Read the model definition and answer for the solid it produces. Units are mm, in the model's axes. Face numbers are marked on the shaded views. A direction names the side the tool comes from. Coordinates: 2 decimals unless noted, no trailing zeros. Loops run counter-clockwise (first coordinate to the right, second up) from the corner with the lowest first, then second, coordinate; pieces in that order, holes last. Notation, with made-up numbers: (85.25, -40) -> (124.25, -40) arc R13 ccw to (124.25, -19) -> close; hole circle Ø3 at (86.5, 37.5). An arc over 180 degrees is marked (long way). Answer in a Markdown table with one row per item.
Autodesk Inventor part; units mm, degrees
ref_plane "YZ Plane" through (0, 0, 0) normal (1, 0, 0) x (0, 1, 0)
ref_plane "XZ Plane" through (0, 0, 0) normal (0, 1, 0) x (-1, 0, 0)
ref_plane "XY Plane" through (0, 0, 0) normal (0, 0, 1) x (1, 0, 0)
sketch "Sketch1" plane through (0, 0, 0) normal (0, 0, 1) x (1, 0, 0)
  circle A0 centre (0, 0) radius 1.5
  dimension "d0" = 3
extrude "Extrusion1" add sketch "Sketch1" along normal blind 5
sketch "Sketch2" plane through (0, 0, 5) normal (0, 0, 1) x (1, 0, 0)
  circle A0 centre (0, 0) radius 1.5
extrude "Extrusion2" add sketch "Sketch2" along normal blind 2 draft 45
sketch "Sketch3" plane through (0, 0, 7) normal (0, 0, 1) x (1, 0, 0)
  circle A0 centre (0, 0) radius 3.5
  circle A1 centre (0, 0) radius 3.35
  dimension "d5" = 6.7
extrude "Extrusion3" cut sketch "Sketch3" against normal blind 2
thread "Thread1"
sketch "Sketch4" plane through (0, 0, 7) normal (0, 0, 1) x (1, 0, 0)
  circle A0 centre (0, 0) radius 3.35
  line L0 (0, -1.1547) -> (-1, -0.5774)
  line L1 (-1, -0.5774) -> (-1, 0.5774)
  line L2 (-1, 0.5774) -> (0, 1.1547)
  line L3 (0, 1.1547) -> (1, 0.5774)
  line L4 (1, 0.5774) -> (1, -0.5774)
  line L5 (1, -0.5774) -> (0, -1.1547)
  dimension "d10" = 1
extrude "Extrusion4" cut sketch "Sketch4" against normal blind 1.5 contours L0 L1 L2 L3 L4 L5
fillet "Fillet1" radius 0.2 6 edges at (-0.5, 0.866, 7) (-1, 0, 7) (-0.5, -0.866, 7) (0.5, -0.866, 7) (1, 0, 7) (0.5, 0.866, 7)
properties part number "bed m3 bolt" material "Stainless Steel"
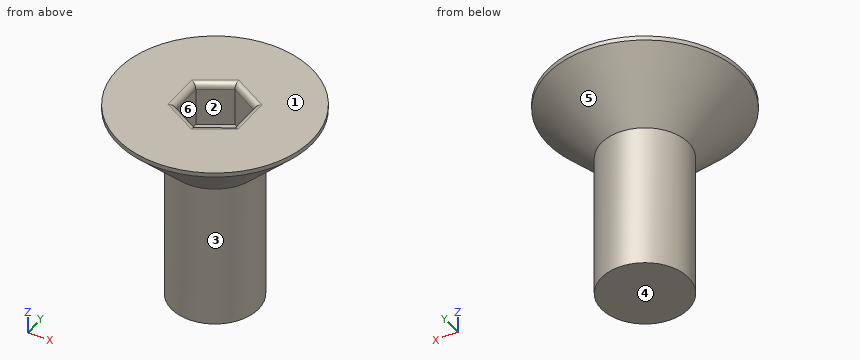
1. Given pin 1 Ø1.5 at (x, z) = (-0.5, 3) entering from +Y; pin 2 Ø4 at (x, z) = (2.5, 3.5) entering from +Y; pin 3 Ø0.9 at (y, z) = (0, 6) entering from +X, each flat-ended and moving along its own axis, determine where each tip first touches the part or whether it passes through.
A:
| item | result |
|---|---|
| pin 1 | stops at y = 1.5 |
| pin 2 | stops at y = 1.41 |
| pin 3 | stops at x = 2.95 |
2. A cutting plane is placed at B-B on z = 3. Give the vertices of the cut face in (x, y).
A:
| item | result |
|---|---|
| outline | circle Ø3 at (0, 0) |
3. The mould has two halves that part along Y. Classify the marked faces 4, 5 and 6: pulls with the +Y half, pulls with the -Y half, needs draft (parallel to the pull), parting line crosses it, or undercut.
A:
| item | result |
|---|---|
| face 4 | needs draft |
| face 5 | parting line crosses it |
| face 6 | undercut |
4. Find the intervals of material crossed by probe 1 along Y at (x, z) = (-0.25, 6.75); probe 2 along Z at (x, y) = (-0.25, 2.5); probe 3 along Y at (x, z) = (0.25, 1), in increasing order.
A:
| item | result |
|---|---|
| probe 1 | y = -3.24 to -1.01, 1.01 to 3.24 |
| probe 2 | z = 6.01 to 7 |
| probe 3 | y = -1.48 to 1.48 |
5. A cutting plane is placed at A-A on y = 0. Give the vertices of the cut face in (x, z).
A:
| item | result |
|---|---|
| outline | (-3.35, 6.85) -> (-1.5, 5) -> (-1.5, 0) -> (1.5, 0) -> (1.5, 5) -> (3.35, 6.85) -> (3.35, 7) -> (1.2, 7) arc R0.2 ccw to (1, 6.8) -> (1, 5.5) -> (-1, 5.5) -> (-1, 6.8) arc R0.2 ccw to (-1.2, 7) -> (-3.35, 7) -> close |
6. A tool of negligible diameter and unlimited length cuts with its end or side. For the marked faces 1, 2 and 3, from which of +Z, -Z, +X, -X, +Y, -Y can it reach the whole face along a straight path? Write none if from no direction.
A:
| item | result |
|---|---|
| face 1 | +Z, +X, -X, +Y, -Y |
| face 2 | +Z |
| face 3 | -Z |
